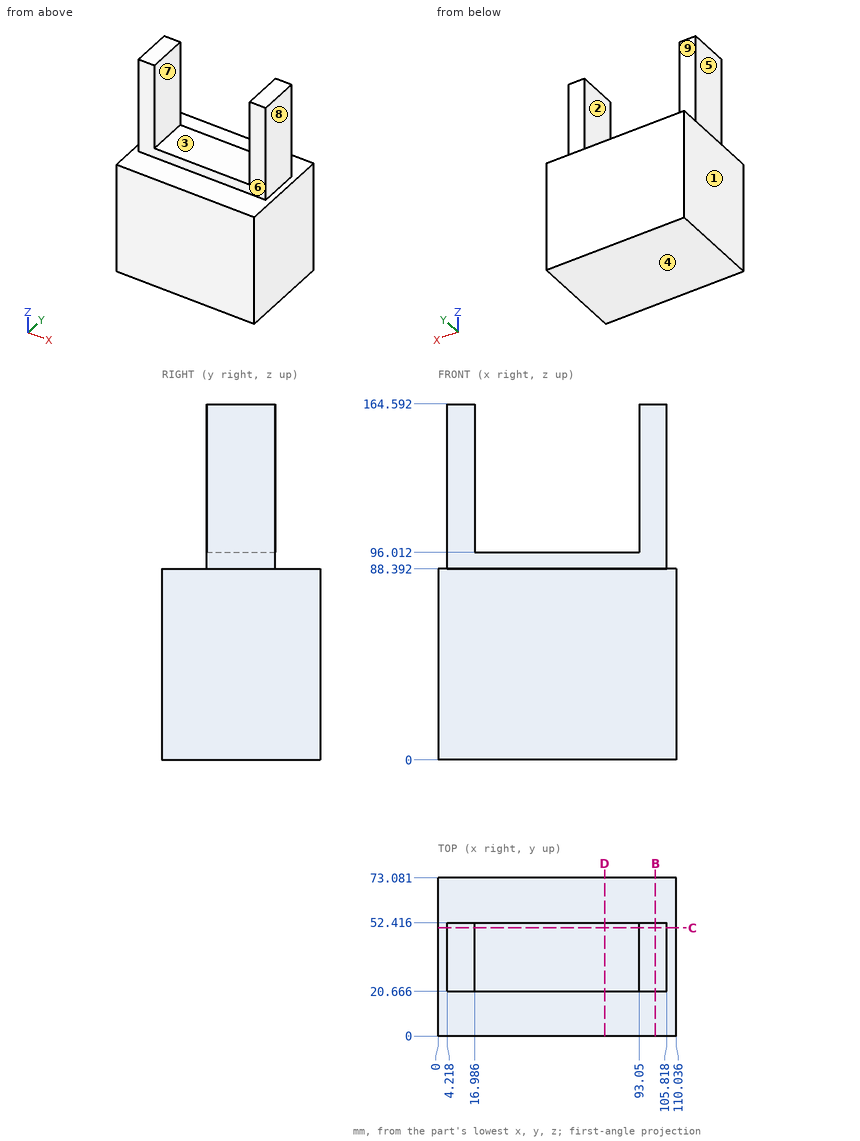
Geometry: see drawing. Coordinates: mm, zero at the bounding-box minimum. A direction names the side the tool comes from. Coordinates: 2 decimals unless noted, no trailing zeros. Order: outer loops, then holes, each group sorted by start corner. A loop starts at its lowest first (then second) coordinate and runs counter-clockwise, first axis right, second up. Notation, with made-up numbers: M 29,-21 L 41,-21 A20 ccw 41,-2 Z; hole C -4.5,18 d4. An arc over 180 degrees is marked long. Write each question's results on one line, items separated by ' | '. Start each with the question number.
1) Contact query for flat-ended pins moving along their axis: pin 1 Ø10 at (y, z) = (40.5, 132) entering from +X; pin 2 Ø6 at (x, z) = (95.5, 127.5) entering from +Y; pin 3 Ø5 at (y, z) = (32, 146) entering from -X. Output: stop coordinate, or through.
2) Draft query along X for the marked faces 1, 2, 3 and 4. Return one class per face: released by +X, released by -X, zero draft, split by the parting line, or undercut.
3) Section query D-D (x = 77). Return the cut outline in (y, z) (1 decimal), plus the area to 3 significant figures.
4) Line query: line 1 (X direction, y = 50, z = 133.5); line 2 (Z direction, x = 37.5, y = 17); line 3 (Z direction, x = 21, y = 36.5). Output: solid intervals per line, ascending. Write a range as from..to.
5) Section query B-B (x = 100.5). Return the cut outline in (y, z) (1 decimal).
6) Section query C-C (y = 50). Return the cut outline in (x, z), plus the area to 3 significant figures.
7) Access query for the marked faces 5, 6, 7, 8 and 9. Directions: +Z, -Z, +X, -X, +Y, -Y. A direction counts if a zero-diameter tool reaches every point of the face in a straight line with its end or side. Return the directions, or none.
Answers:
1) pin 1: stops at x = 105.82 | pin 2: stops at y = 52.42 | pin 3: stops at x = 4.22
2) face 1: released by -X | face 2: undercut | face 3: undercut | face 4: zero draft
3) outline: M 0,0 L 73.1,0 L 73.1,88.4 L 52.4,88.4 L 52.4,96 L 20.7,96 L 20.7,88.4 L 0,88.4 Z | area: 6,700 mm^2
4) line 1: x = 4.22..16.99, 93.05..105.82 | line 2: z = 0..88.39 | line 3: z = 0..96.01
5) outline: M 0,0 L 73.1,0 L 73.1,88.4 L 52.4,88.4 L 52.4,164.6 L 20.7,164.6 L 20.7,88.4 L 0,88.4 Z
6) outline: M 0,0 L 110.04,0 L 110.04,88.39 L 105.82,88.39 L 105.82,164.59 L 93.05,164.59 L 93.05,96.01 L 16.99,96.01 L 16.99,164.59 L 4.22,164.59 L 4.22,88.39 L 0,88.39 Z | area: 12,300 mm^2
7) face 5: +Z, -X, +Y, -Y | face 6: +Z, +X, -X, -Y | face 7: +Z, +Y, -Y | face 8: +Z, +X, +Y, -Y | face 9: +Z, +X, -X, +Y
